from build123d import *

# Parameters (mm, degrees)
SKETCH_1_W          = 15
SKETCH_1_H          = 15
SKETCH_1_W_2        = 13
SKETCH_1_H_2        = 13
EXTRUDE_1_DEPTH     = 270
SKETCH_2_R          = 1.5
SKETCH_2_R_2        = 2.5
CUT_EXTRUDE_1_DEPTH = 271.520331953
SKETCH_3_R          = 1.5
CUT_EXTRUDE_2_DEPTH = 271.520331953


with BuildPart() as part:
    # 草图1 → 凸台-拉伸1 (new body)
    with BuildSketch(Plane(origin=(0, 0, 0), x_dir=(1, 0, 0), z_dir=(0, 1, 0))):
        Rectangle(SKETCH_1_W, SKETCH_1_H)
        Rectangle(SKETCH_1_W_2, SKETCH_1_H_2, mode=Mode.SUBTRACT)
    extrude(amount=EXTRUDE_1_DEPTH)

    # 草图2 → 切除-拉伸1 (cut, through all)
    with BuildSketch(Plane.XY.offset(7.5)):
        with Locations((0, 155)):
            Circle(SKETCH_2_R)
        with Locations((0, 115)):
            Circle(SKETCH_2_R)
        with Locations((0, 200)):
            Circle(SKETCH_2_R)
        with Locations((0, 70)):
            Circle(SKETCH_2_R)
        with Locations((0, 220)):
            Circle(SKETCH_2_R_2)
        with Locations((0, 50)):
            Circle(SKETCH_2_R_2)
    extrude(amount=-CUT_EXTRUDE_1_DEPTH, mode=Mode.SUBTRACT)

    # 草图3 → 切除-拉伸2 (cut, through all)
    with BuildSketch(Plane(origin=(7.5, 0, 0), x_dir=(0, 0, -1), z_dir=(1, 0, 0))):
        with Locations((0, 240)):
            Circle(SKETCH_3_R)
        with Locations((0, 30)):
            Circle(SKETCH_3_R)
        with Locations((0, 10)):
            Circle(SKETCH_3_R)
        with Locations((0, 260)):
            Circle(SKETCH_3_R)
    extrude(amount=-CUT_EXTRUDE_2_DEPTH, mode=Mode.SUBTRACT)


solid = part.part
Input: part model. Units: mm. Frame: model coordinates. A direction names the side the tool comes from. Coordinates: 2 decimals unless noted, no trailing zeros. Loops run counter-clockwise (first coordinate to the right, second up) from the corner with the lowest first, then second, coordinate; pieces in that order, holes last. Notation, with made-up numbers: (-37.5, -19) -> (9.5, -19) arc R20 cw to (9.5, 14) -> close; hole circle Ø3 at (78, 15). An arc over 180 degrees is marked (long way). Write each question's results on one line, items separated by ' | '. Start each with the question number.
Q1. Section B-B, the plane y = 162. Return the cut outline in (x, z).
Q2. Reachability of faces 4 (the flat face through (0, 133, 6.5)), 5 (the flat face through (0, 133, -7.5)) from +Z, -Z, +X, -X, +Y, -Y: full face, straight path, thin tool, end or side. Return the list, or none.
Q3. Pin query (flat end, axial travel): pin 1 (2.5 mm diameter, centred on y = 10, z = 0, fed in from -X) (3 decimals). Return the tip coordinate at first contact, or that it passes through.
Q4. Pull-direction query (Y, two-part tool) for faces 1 (the flat face through (0, 133, -6.5)), 2 (the flat face through (-7, 270, 0)), 3 (the cylindrical face through (-0.33, 222.48, -6.99)); classes: released by +Y, released by -Y, zero draft, split by the parting line, or undercut.
Q5. Ray query, line 1 (Y direction, x = 7.05, z = 0); line 2 (Z direction, x = 1.75, y = 217). Return the intervals inside material, ascending. Write a range as from..to.
Q6. Section A-A, the plane y = 50. Return the cut outline in (x, z), plus the area to 3 significant figures.
Found:
1) outline: (-7.5, -7.5) -> (7.5, -7.5) -> (7.5, 7.5) -> (-7.5, 7.5) -> close; hole (-6.5, -6.5) -> (6.5, -6.5) -> (6.5, 6.5) -> (-6.5, 6.5) -> close
2) face 4: +Y, -Y | face 5: -Z, +X, -X, +Y, -Y
3) pin 1: through
4) face 1: zero draft | face 2: released by +Y | face 3: undercut
5) line 1: 0..8.5, 11.5..28.5, 31.5..238.5, 241.5..258.5, 261.5..270 | line 2: -7.5..-6.5, 6.5..7.5
6) outline: (-7.5, -7.5) -> (-2.5, -7.5) -> (-2.5, -6.5) -> (-6.5, -6.5) -> (-6.5, 6.5) -> (-2.5, 6.5) -> (-2.5, 7.5) -> (-7.5, 7.5) -> close; (2.5, -7.5) -> (7.5, -7.5) -> (7.5, 7.5) -> (2.5, 7.5) -> (2.5, 6.5) -> (6.5, 6.5) -> (6.5, -6.5) -> (2.5, -6.5) -> close | area: 46.0 mm2
